Job drawing, mm, ordinate dimensions from the low corner. One solid piece. A direction names the side the tool comes from. Give positions to 0.01 mm unless a question says otherwise; leave off trailing zeros. Order: outer loops, then holes, each group sorted by start corner. A loop starts at its lowest first (then second) coordinate and runs counter-clockwise, first axis right, second up. Notation, with made-up numbers: (52.5, 66) -> (90.5, 66) arc R29 cw to (90.5, 98) -> close; hole circle Ø3 at (68, 47.5). An arc over 180 degrees is marked (long way). Write item = value, one per line. Start each with the question number.
(1) Saw through at D-D, the plane z = 4.5. List the corners of the cut face in (x, y), then the cut area to 3 significant figures.
(2) Flat gauge pins, fed straight in: pin 1 (1.5 mm diameter, centred on x = 12.5, z = 13.5, fed in from -Y); pin 2 (0.7 mm diameter, centred on x = 10.5, y = 18, fed in from +Z); pin 3 (2 mm diameter, centred on y = 14.5, z = 6.5, fed in from -X). Where does each tip first touch, or does it go through?
(3) Saw through at A-A, the plane y = 13.25. List the corners of the cut face in (x, z) (1 decimal), then the cut area to 3 significant figures.
(4) Saw through at B-B, the plane x = 6. List the corners of the cut face in (y, z) (1 decimal).
(5) Two-plate mould, pull along X, no slides. Class the marked faces 1, 2, 3 and 4: pulls with the +X half, pulls with the -X half, needs draft (parallel to the pull), parting line crosses it, or undercut.
(6) Probe line 1 along Y through (x, z) = (10, 6); line 2 along X through (y, z) = (10.5, 16.5); line 3 along X through (y, z) = (10.25, 7.5). List the from-to ranges inside material, lowest first. Write a range as from..to.
(7) Which spindle directions (+Z, -Z, +X, -X, +Y, -Y) get a long thin tool onto all of the face, cutting with end or side? Do the marked faces 5 and 6. Say none if no direction does.
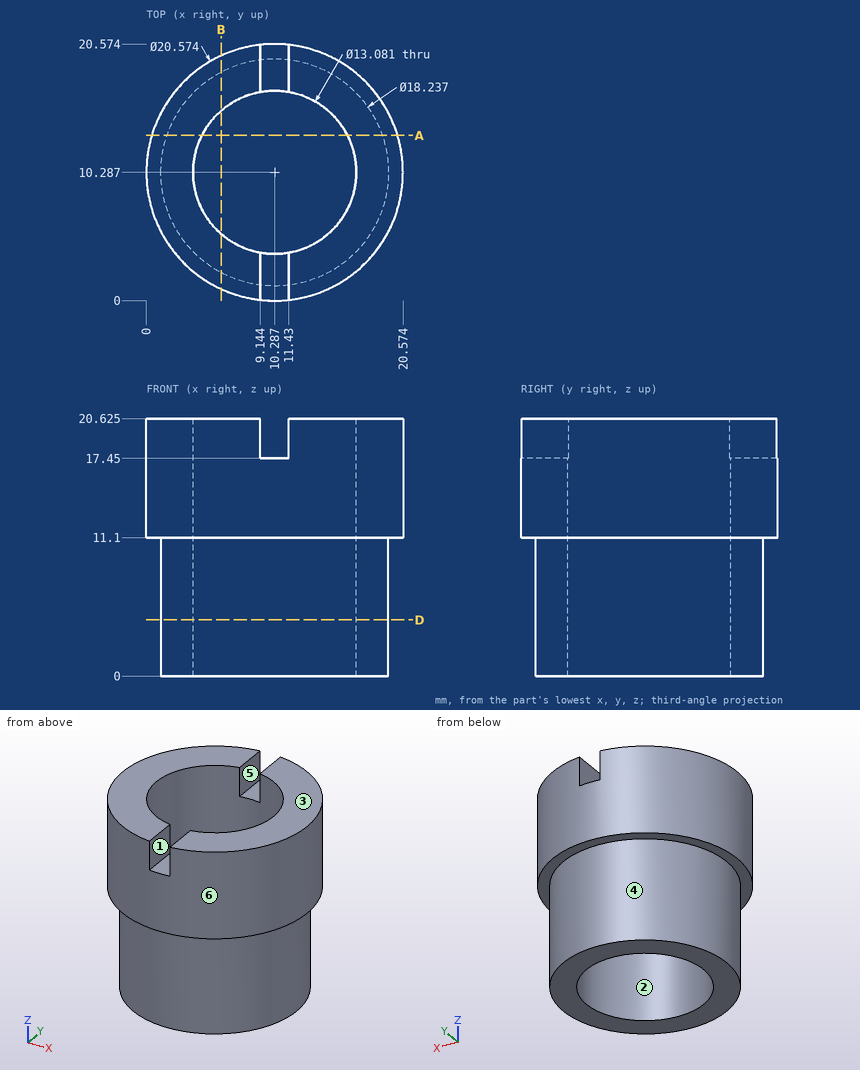
Results list:
q1.outline = circle Ø18.24 at (10.29, 10.29); hole circle Ø13.08 at (10.29, 10.29)
q1.area = 127 mm^2
q2.pin_1 = 0.1
q2.pin_2 = 17.45
q2.pin_3 = 1.75
q3.outline = (0.4, 11.1) -> (1.7, 11.1) -> (1.7, 0) -> (4.5, 0) -> (4.5, 20.6) -> (0.4, 20.6) -> close; (16.1, 0) -> (18.9, 0) -> (18.9, 11.1) -> (20.1, 11.1) -> (20.1, 20.6) -> (16.1, 20.6) -> close
q3.area = 139 mm^2
q4.outline = (0.9, 11.1) -> (2.2, 11.1) -> (2.2, 0) -> (5.3, 0) -> (5.3, 20.6) -> (0.9, 20.6) -> close; (15.2, 0) -> (18.3, 0) -> (18.3, 11.1) -> (19.6, 11.1) -> (19.6, 20.6) -> (15.2, 20.6) -> close
q5.face_1 = undercut
q5.face_2 = undercut
q5.face_3 = needs draft
q5.face_4 = parting line crosses it
q6.line_1 = 1.17..3.75, 16.82..19.4
q6.line_2 = 0..3.75, 16.82..20.57
q6.line_3 = 1.17..3.75, 16.83..19.41
q7.face_5 = +Z, +Y, -Y
q7.face_6 = +Z, -Z
